Check sheet for the modelled part. Datum: model origin and axes. Units: mm. A direction names the side the tool comes from. Give positions to 0.01 mm unless a question says otherwise; leave off trailing zeros. Write each loop counter-clockwise with the first axis right and the second up, starting at its lowest first coordinate (ties: lowest second). Pieces come first, ordered by that corner, then holes.
from build123d import *

# Parameters (mm, degrees)
SKETCH2_R           = 14.2875
SKETCH2_R_2         = 19.05
SKETCH2_R_3         = 5.0419
SKETCH2_R_4         = 3.3782
SKETCH2_R_5         = 5.08
SKETCH2_R_6         = 2.5527
BOSS_EXTRUDE1_DEPTH = 5.588
SKETCH4_R           = 2.5527
CUT_EXTRUDE1_DEPTH  = 6.588
SKETCH6_R           = 1.651
CUT_EXTRUDE2_DEPTH  = 6.588


with BuildPart() as part:
    # Sketch2 → Boss-Extrude1 (new body)
    with BuildSketch(Plane(origin=(0, 0, 0), x_dir=(0, 0, -1), z_dir=(1, 0, 0))):
        with BuildLine():
            Line((-444.051224287, -73.655160045), (-452.990991726, 20.219177))
            ThreePointArc((-452.990991726, 20.219177), (-459.828166258, 38.628688745), (-474.92551535, 51.187634905))
            ThreePointArc((-474.92551535, 51.187634905), (-482.292216482, 62.940162968), (-474.512475698, 74.423447984))
            Line((-474.512475698, 74.423447984), (-242.526195837, 171.867023314))
            ThreePointArc((-242.526195837, 171.867023314), (-227.371894365, 174.215557577), (-212.884484768, 169.18729451))
            Line((-212.884484768, 169.18729451), (13.876862492, 21.274225894))
            ThreePointArc((13.876862492, 21.274225894), (25.333435416, -1.837675174), (10.661298989, -23.05421228))
            Line((10.661298989, -23.05421228), (-53.518911784, -52.734012568))
            ThreePointArc((-53.518911784, -52.734012568), (-59.768398865, -53.873624135), (-65.787992524, -51.844019374))
            Line((-65.787992524, -51.844019374), (-152.593044897, 4.777630757))
            ThreePointArc((-152.593044897, 4.777630757), (-288.489875105, 20.154119165), (-381.997670333, -79.649072608))
            ThreePointArc((-381.997670333, -79.649072608), (-415.496829233, -102.248099493), (-444.051224287, -73.655160045))
        make_face()
        with Locations((-230.230562883, 142.594512143)):
            Circle(SKETCH2_R, mode=Mode.SUBTRACT)
        with Locations((-353.440471878, 63.406794563)):
            Circle(SKETCH2_R, mode=Mode.SUBTRACT)
        with Locations((-412.444222517, -70.645186775)):
            Circle(SKETCH2_R, mode=Mode.SUBTRACT)
        with Locations((-425.144222517, 62.714443515)):
            Circle(SKETCH2_R_2, mode=Mode.SUBTRACT)
        Circle(SKETCH2_R_3, mode=Mode.SUBTRACT)
        with Locations((-58.849561279, -41.206906428)):
            Circle(SKETCH2_R_4, mode=Mode.SUBTRACT)
        with Locations((-267.623520866, 118.561842852)):
            Circle(SKETCH2_R_4, mode=Mode.SUBTRACT)
        with Locations((-407.183710275, 80.674955757)):
            Circle(SKETCH2_R_5, mode=Mode.SUBTRACT)
        with Locations((-443.104734759, 80.674955757)):
            Circle(SKETCH2_R_6, mode=Mode.SUBTRACT)
        with Locations((-443.104734759, 44.753931273)):
            Circle(SKETCH2_R_5, mode=Mode.SUBTRACT)
        with Locations((-407.183710275, 44.753931273)):
            Circle(SKETCH2_R_6, mode=Mode.SUBTRACT)
        with Locations((-469.594222517, 62.714443515)):
            Circle(SKETCH2_R_4, mode=Mode.SUBTRACT)
        with Locations((-431.494222517, -13.485556485)):
            Circle(SKETCH2_R_4, mode=Mode.SUBTRACT)
        with Locations((-380.694222517, 94.464443515)):
            Circle(SKETCH2_R_4, mode=Mode.SUBTRACT)
    extrude(amount=BOSS_EXTRUDE1_DEPTH)

    # Sketch4 → Cut-Extrude1 (cut, through all)
    with BuildSketch(Plane(origin=(5.588, 0, 0), x_dir=(0, 0, -1), z_dir=(1, 0, 0))):
        with Locations((-293.761614403, 143.45865083)):
            Circle(SKETCH4_R)
        with Locations((-152.53102271, 122.238150561)):
            Circle(SKETCH4_R)
        with Locations((-53.415030813, 57.586256896)):
            Circle(SKETCH4_R)
    extrude(amount=-CUT_EXTRUDE1_DEPTH, mode=Mode.SUBTRACT)

    # Sketch6 → Cut-Extrude2 (cut, through all)
    with BuildSketch(Plane(origin=(5.588, 0, 0), x_dir=(0, 0, -1), z_dir=(1, 0, 0))):
        with Locations((-17.434256382, 26.535056141)):
            Circle(SKETCH6_R)
        with Locations((-159.544838365, 23.538860962)):
            Circle(SKETCH6_R)
        with Locations((-77.805734295, 65.914477118)):
            Circle(SKETCH6_R)
        with Locations((-245.562662209, 41.946583471)):
            Circle(SKETCH6_R)
        with Locations((-261.025951592, 150.321512483)):
            Circle(SKETCH6_R)
        with Locations((-328.824486777, 13.567386224)):
            Circle(SKETCH6_R)
        with Locations((-385.694231257, -53.542541728)):
            Circle(SKETCH6_R)
        with Locations((-439.565263827, 13.201837119)):
            Circle(SKETCH6_R)
        with Locations((-314.936803191, 127.67678482)):
            Circle(SKETCH6_R)
        with Locations((-368.84765479, 105.032057158)):
            Circle(SKETCH6_R)
        with Locations((-138.177212208, 105.293898095)):
            Circle(SKETCH6_R)
        with Locations((-85.442343646, -23.860828313)):
            Circle(SKETCH6_R)
        with Locations((-433.816402195, -47.165569321)):
            Circle(SKETCH6_R)
        with Locations((-198.54869012, 144.673319072)):
            Circle(SKETCH6_R)
        with Locations((-234.184271033, 98.860730407)):
            Circle(SKETCH6_R)
        with Locations((-384.29522028, 43.783484838)):
            Circle(SKETCH6_R)
        with Locations((-311.243516345, 76.78330883)):
            Circle(SKETCH6_R)
        with Locations((-184.277438268, 73.672869391)):
            Circle(SKETCH6_R)
        with Locations((-100.025478144, 34.964630862)):
            Circle(SKETCH6_R)
    extrude(amount=-CUT_EXTRUDE2_DEPTH, mode=Mode.SUBTRACT)


solid = part.part
1) Sectioned sample at A-A on z = 420.5. Record the boundary of the cut face in (x, y).
2) Draft check along Y on faces 3 (the flat face through (5.588, 38, 281)), 4 (the flat face through (2.755, -37.686, 20.98)), 5 (the cylindrical face through (2.755, 48.187, 446.849)). Enter one of: +Y half, -Y half, draft (parallel to the pull), parting line (faces both ways), or undercut.
3) Gauge pin test, flat ends, axial feed: pin 1 (2.5 mm diameter, centred on y = 105.29, z = 138.18, fed in from +X); pin 2 (1 mm diameter, centred on x = 3, y = 24, fed in from -Z); pin 3 (1 mm diameter, centred on x = 1, z = 170.5, fed in from -Y); pin 4 (3 mm diameter, centred on x = 4, y = 141.5, fed in from +Z). Record the tip position at first contact, or that the pin passes through.
4) Sectioned sample at B-B on y = 0. Record the boundary of the cut face in (x, z), then the cut area to 3 significant figures.
5) Access from +Z, -Z, +X, -X, +Y, -Y to the whole of each face (thin tool, end or side, straight path). Record for faces 1 (the cylindrical face through (2.755, 68.437, 406.974)), 2 (the flat face through (2.75, -23.93, 108.58)).
6) Scan lines: L1, parallel to Z at x = 2, y = -47; L2, parallel to Z at x = 3, y = 65; L3, parallel to Z at x = 1.5, y = 80. Record each from-to range of solid material in increasing order.
7) Sectioned sample at C-C on z = 0. Record the boundary of the cut face in (x, y).
8) Sectioned sample at D-D on x = 1.7. Give the number of separate pieces and of enclosed holes in the cut face, then the cut area to 3 significant figures.
Answers below:
1. outline: (0, -101.36) - (5.59, -101.36) - (5.59, -82.45) - (0, -82.45) - close; (0, -58.85) - (5.59, -58.85) - (5.59, 44.24) - (0, 44.24) - close; (0, 81.19) - (5.59, 81.19) - (5.59, 97.11) - (0, 97.11) - close
2. face 3: draft
2. face 4: -Y half
2. face 5: undercut
3. pin 1: passes through
3. pin 2: stops at z = -10.46
3. pin 3: stops at y = 14.57
3. pin 4: stops at z = 318.39
4. outline: (0, -25.4) - (5.59, -25.4) - (5.59, -5.04) - (0, -5.04) - close; (0, 5.04) - (5.59, 5.04) - (5.59, 145.27) - (0, 145.27) - close; (0, 326.02) - (5.59, 326.02) - (5.59, 451.07) - (0, 451.07) - close
4. area: 1,600 mm2
5. face 1: +X, -X
5. face 2: +X, -X, -Y
6. L1: z = 41.12 to 73.21, 368.03 to 432.17, 435.46 to 446.59
6. L2: z = 53.16 to 76.43, 79.18 to 339.24, 367.64 to 406.23, 444.06 to 467.11, 472.08 to 482.09
6. L3: z = 76.15 to 402.15, 412.22 to 417.14, 433.15 to 440.64, 445.57 to 461.24
7. outline: (0, -27.98) - (5.59, -27.98) - (5.59, -5.04) - (0, -5.04) - close; (0, 5.04) - (5.59, 5.04) - (5.59, 30.33) - (0, 30.33) - close
8. separate pieces: 1
8. enclosed holes: 36
8. area: 60,600 mm2
